from build123d import *

# Parameters (mm, degrees)
SKETCH_1_W              = 430
SKETCH_1_H              = 245
EXTRUDE_1_DEPTH         = 6
SKETCH_2_R              = 22.5
CUT_EXTRUDE_1_DEPTH     = 13
HOLE_WIZARD_M6_1_D      = 5
CUT_EXTRUDE_2_DEPTH     = 13
HOLE_WIZARD_13_0_13_1_D = 13
CUT_EXTRUDE_3_DEPTH     = 13
EXTRUDE_2_DEPTH         = 12
FILLET_1_R              = 10
SKETCH_11_R             = 30
CUT_EXTRUDE_4_DEPTH     = 13
HOLE_WIZARD_11_0_11_1_D = 11


with BuildPart() as part:
    # 草图1 → 凸台-拉伸1 (new body, symmetric)
    with BuildSketch(Plane.XY):
        Rectangle(SKETCH_1_W, SKETCH_1_H)
    extrude(amount=EXTRUDE_1_DEPTH, both=True)

    # 草图2 → 切除-拉伸1 (cut, through all)
    with BuildSketch(Plane.XY.offset(6)):
        with Locations((-175, 87.5)):
            Circle(SKETCH_2_R)
        with Locations((175, 87.5)):
            Circle(SKETCH_2_R)
        with Locations((175, -87.5)):
            Circle(SKETCH_2_R)
        with Locations((-175, -87.5)):
            Circle(SKETCH_2_R)
    extrude(amount=-CUT_EXTRUDE_1_DEPTH, mode=Mode.SUBTRACT)

    # M6 螺纹孔1 (through all)
    with Locations(Plane.XY.offset(6)):
        with Locations((-199.5, 105), (-150.5, 105), (-150.5, 70), (-199.5, 70), (199.5, 70), (150.5, 70), (150.5, 105), (199.5, 105), (199.5, -105), (150.5, -105), (150.5, -70), (199.5, -70), (-199.5, -70), (-150.5, -70), (-150.5, -105), (-199.5, -105)):
            Hole(HOLE_WIZARD_M6_1_D / 2)

    # 草图5 → 切除-拉伸2 (cut, through all)
    with BuildSketch(Plane.XY.offset(6)):
        with BuildLine():
            Line((-130, -70), (130, -70))
            ThreePointArc((130, -70), (137.071067812, -67.071067812), (140, -60))
            Line((140, -60), (140, 60))
            ThreePointArc((140, 60), (137.071067812, 67.071067812), (130, 70))
            Line((130, 70), (-130, 70))
            ThreePointArc((-130, 70), (-137.071067812, 67.071067812), (-140, 60))
            Line((-140, 60), (-140, -60))
            ThreePointArc((-140, -60), (-137.071067812, -67.071067812), (-130, -70))
        make_face()
    extrude(amount=-CUT_EXTRUDE_2_DEPTH, mode=Mode.SUBTRACT)

    # Ø13.0 (13) 直径孔1 (through all)
    with Locations(Plane(origin=(0, 0, -6), x_dir=(-1, 0, 0), z_dir=(0, 0, -1))):
        with Locations((-110, 87.5), (110, 87.5), (110, -87.5), (-110, -87.5)):
            Hole(HOLE_WIZARD_13_0_13_1_D / 2)

    # 草图8 → 切除-拉伸3 (cut, through all)
    with BuildSketch(Plane(origin=(0, 0, -6), x_dir=(-1, 0, 0), z_dir=(0, 0, -1))):
        with BuildLine():
            Line((-80, 70), (80, 70))
            Line((80, 70), (80, 95))
            ThreePointArc((80, 95), (77.071067812, 102.071067812), (70, 105))
            Line((70, 105), (-70, 105))
            ThreePointArc((-70, 105), (-77.071067812, 102.071067812), (-80, 95))
            Line((-80, 95), (-80, 70))
        make_face()
        with BuildLine():
            Line((80, -70), (80, -95))
            ThreePointArc((80, -95), (77.071067812, -102.071067812), (70, -105))
            Line((70, -105), (-70, -105))
            ThreePointArc((-70, -105), (-77.071067812, -102.071067812), (-80, -95))
            Line((-80, -95), (-80, -70))
            Line((-80, -70), (80, -70))
        make_face()
    extrude(amount=-CUT_EXTRUDE_3_DEPTH, mode=Mode.SUBTRACT)

    # 草图10 → 凸台-拉伸2 (add)
    with BuildSketch(Plane(origin=(0, 0, -6), x_dir=(-1, 0, 0), z_dir=(0, 0, -1))):
        with BuildLine():
            Line((-80, -70), (-80, -95))
            ThreePointArc((-80, -95), (-77.071067812, -102.071067812), (-70, -105))
            Line((-70, -105), (70, -105))
            ThreePointArc((70, -105), (77.071067812, -102.071067812), (80, -95))
            Line((80, -95), (80, -70))
            Line((80, -70), (80, 70))
            Line((80, 70), (80, 95))
            ThreePointArc((80, 95), (77.071067812, 102.071067812), (70, 105))
            Line((70, 105), (-70, 105))
            ThreePointArc((-70, 105), (-77.071067812, 102.071067812), (-80, 95))
            Line((-80, 95), (-80, 70))
            Line((-80, 70), (-80, -70))
        make_face()
    extrude(amount=-EXTRUDE_2_DEPTH)

    # 圆角1
    fillet_1_edges = [part.edges().sort_by_distance(p)[0] for p in [
        (80, 70, 0),
        (-80, 70, 0),
        (80, -70, 0),
        (-80, -70, 0),
    ]]
    fillet(fillet_1_edges, radius=FILLET_1_R)

    # 草图11 → 切除-拉伸4 (cut, through all)
    with BuildSketch(Plane(origin=(0, 0, -6), x_dir=(-1, 0, 0), z_dir=(0, 0, -1))):
        Circle(SKETCH_11_R)
    extrude(amount=-CUT_EXTRUDE_4_DEPTH, mode=Mode.SUBTRACT)

    # Ø11.0 (11) 直径孔1 (through all)
    with Locations(Plane(origin=(44.5, 44.5, -6), x_dir=(-1, 0, 0), z_dir=(0, 0, -1))):
        with Locations((0, 0), (89, 0), (89, -89), (0, -89)):
            Hole(HOLE_WIZARD_11_0_11_1_D / 2)


solid = part.part
Source: CAD feature listing. Evaluate the final solid. Frame: model axes, mm. A direction names the side the tool comes from. Coordinates: 2 decimals unless noted, no trailing zeros. Loops run counter-clockwise (first coordinate to the right, second up) from the corner with the lowest first, then second, coordinate; pieces in that order, holes last. Notation, with made-up numbers: (64, 34) - (98, 34) arc R7 ccw to (98, 42) - close; hole circle Ø5 at (6.25, -13.5). An arc over 180 degrees is marked (long way). One line per question, with ' | ' between items.
1) Section D-D, the plane y = 0. Return loops of the section in (x, z), then the cut area to 3 significant figures.
Report:
outline: (-215, -6) - (-140, -6) - (-140, 6) - (-215, 6) - close; (-80, -6) - (-30, -6) - (-30, 6) - (-80, 6) - close; (30, -6) - (80, -6) - (80, 6) - (30, 6) - close; (140, -6) - (215, -6) - (215, 6) - (140, 6) - close | area: 3,000 mm²
2) Section B-B, the plane y = -87.5. Return loops of the section in (x, z).
Report:
outline: (-215, -6) - (-197.5, -6) - (-197.5, 6) - (-215, 6) - close; (-152.5, -6) - (-116.5, -6) - (-116.5, 6) - (-152.5, 6) - close; (-103.5, -6) - (103.5, -6) - (103.5, 6) - (-103.5, 6) - close; (116.5, -6) - (152.5, -6) - (152.5, 6) - (116.5, 6) - close; (197.5, -6) - (215, -6) - (215, 6) - (197.5, 6) - close
3) Set-up query: faces 1 (the face through (80, 1, 0)), 2 (the face through (-3, 122.5, 0)). Return all of +Z, -Z, +X, -X, +Y, -Y with unobstructed straight access to the full face (end or side cutting, diameter ignored); none if empty.
Report:
face 1: +Z, -Z | face 2: +Z, -Z, +X, -X, +Y
4) Section A-A, the plane x = -175. Return loops of the section in (y, z).
Report:
outline: (-122.5, -6) - (-110, -6) - (-110, 6) - (-122.5, 6) - close; (-65, -6) - (65, -6) - (65, 6) - (-65, 6) - close; (110, -6) - (122.5, -6) - (122.5, 6) - (110, 6) - close
5) Pull-direction query (X, two-part tool) for faces 3 (the face through (140, -1, 0)), 4 (the face through (-215, -2, 0)), 5 (the face through (-110, 70, 0)), 6 (the face through (51, 2, -6)); classes: released by +X, released by -X, zero draft, split by the parting line, or undercut.
Report:
face 3: undercut | face 4: released by -X | face 5: undercut | face 6: zero draft
6) Section C-C, the plane x = -110. Return loops of the section in (y, z), then the cut area to 3 significant figures.
Report:
outline: (-122.5, -6) - (-94, -6) - (-94, 6) - (-122.5, 6) - close; (-81, -6) - (-70, -6) - (-70, 6) - (-81, 6) - close; (70, -6) - (81, -6) - (81, 6) - (70, 6) - close; (94, -6) - (122.5, -6) - (122.5, 6) - (94, 6) - close | area: 948 mm²
7) Line query: line 1 along Y through (x, z) = (-199.5, 2.5); line 2 along Y through (x, z) = (175, 0); line 3 along X through (y, z) = (60, -1.25). Output: solid intervals per line, ascending.
Report:
line 1: y = -122.5 to -107.5, -102.5 to -72.5, -67.5 to 67.5, 72.5 to 102.5, 107.5 to 122.5 | line 2: y = -122.5 to -110, -65 to 65, 110 to 122.5 | line 3: x = -215 to -140, -80 to 80, 140 to 215
